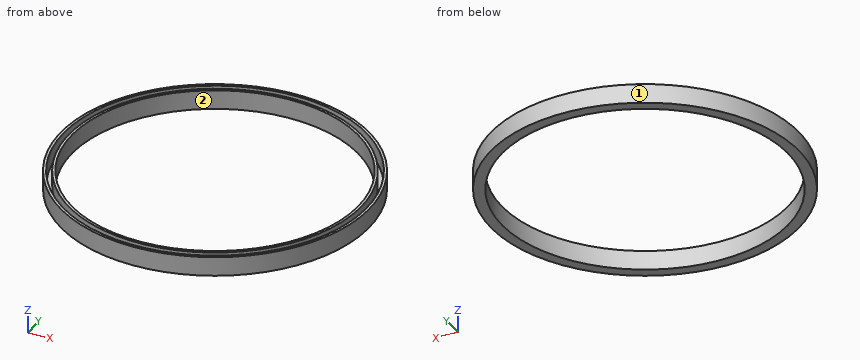
from build123d import *

# Parameters (mm, degrees)
F0_R     = 28
F0_R_2   = 27.5
F0_R_3   = 26.5
F0_R_4   = 26
F1_DEPTH = 3
F2_R     = 28
F2_R_2   = 26
F3_DEPTH = 0.5


with BuildPart() as f1:
    # F0 (on Top) → F1 (new body)
    with BuildSketch(Plane.XY):
        Circle(F0_R)
        Circle(F0_R_2, mode=Mode.SUBTRACT)
        Circle(F0_R_3)
        Circle(F0_R_4, mode=Mode.SUBTRACT)
    extrude(amount=F1_DEPTH)

    # F2 (on face) → F3 (join)
    with BuildSketch(Plane(origin=(0, 0, 0), x_dir=(1, 0, 0), z_dir=(0, 0, -1))):
        Circle(F2_R)
        Circle(F2_R_2, mode=Mode.SUBTRACT)
    extrude(amount=F3_DEPTH)


solid = f1.part
Check sheet for the modelled part. Datum: model origin and axes. Units: mm. Face numbers are marked on the shaded views. Give positions to 0.01 mm unless a question says otherwise; leave off trailing zeros. Loops run counter-clockwise (first coordinate to the right, second up) from the corner with the lowest first, then second, coordinate; pieces in that order, holes last. Notation, with made-up numbers: M 46.5,54.25 L 86.5,54.25 A17 cw 86.5,63.25 Z; hole C 15.5,8 d2. An arc over 180 degrees is marked long. Answer as a JSON object with one key per item and string values. Group by question number.
Q1. Go/stop test with flat-tipped pins: P1, Ø2, axis at x = 0.5, z = 1.5, coming from the +Y side; P2, Ø1, axis at y = -2.5, z = 0.5, coming from the +X side. Record where each tip stops, or that it passes through.
Q2. Cross-section at A-A on y = 0. Record the cut outline in (x, z), then the cut area to 3 significant figures.
Q3. Release check for a two-part mould opening along Y. For the marked faces 1 and 2 record: released by +Y, released by -Y, zero draft, split by the parting line, or undercut.
Q4. Cross-section at C-C on z = 0.6. Record the cut outline in (x, y), then the cut area to 3 significant figures.
Q5. Material ranges on line 1 along Y through (x, z) = (0, 2.15); line 2 along X through (y, z) = (-4, 2.85); line 3 along Y through (x, z) = (18, 0.9), recorded low to high. Write a range as [from, to].
Evaluation:
{
 "1": {"P1": "stops at y = 28", "P2": "stops at x = 27.93"},
 "2": {"outline": "M -28,-0.5 L -26,-0.5 L -26,3 L -26.5,3 L -26.5,0 L -27.5,0 L -27.5,3 L -28,3 Z; M 26,-0.5 L 28,-0.5 L 28,3 L 27.5,3 L 27.5,0 L 26.5,0 L 26.5,3 L 26,3 Z", "area": "8.00 mm2"},
 "3": {"face 1": "split by the parting line", "face 2": "undercut"},
 "4": {"outline": "C 0,0 d56; C 0,0 d53; hole C 0,0 d55; hole C 0,0 d52", "area": "170 mm2"},
 "5": {"line 1": "y = [-28, -27.5], [-26.5, -26], [26, 26.5], [27.5, 28]", "line 2": "x = [-27.71, -27.21], [-26.2, -25.69], [25.69, 26.2], [27.21, 27.71]", "line 3": "y = [-21.45, -20.79], [-19.45, -18.76], [18.76, 19.45], [20.79, 21.45]"}
}
